The figure shows three views and two pictorial views of one solid part (mm, origin at its lowest corner). Answer the questions. A direction names the side the tool comes from. Round coordinates to 2 decimals unless told otherwise and drop trailing zeros. Order: outer loops, then holes, each group sorted by start corner. A loop starts at its lowest first (then second) coordinate and runs counter-clockwise, first axis right, second up. Notation, with made-up numbers: (26.5, 69.25) - (73.5, 69.25) arc R21 ccw to (73.5, 102.25) - close; hole circle Ø2 at (12, 81). An arc over 180 degrees is marked (long way). One line per item, written item: value. Start each with the question number.
1. Section C-C, the plane x = 17 is taken. Give the vertices of the cut face in (y, z), then the cut area to 3 significant figures.
2. Section D-D, the plane y = 12 is taken. Give the vertices of the cut face in (x, z).
3. For a pull along Y with two mould halves and no side action, classify the marked faces 3, 4, 5 and 6 as released by +Y, released by -Y, zero draft, split by the parting line, or undercut.
4. Flat-ended cylindrical pins translate along their axes: P1, Ø6, axis at x = 10, y = 7.5, coming from the +Z side; P2, Ø1.5, axis at y = 2.5, z = 7, coming from the +X side. Find the tip coordinate at first contact, or state that the pin passes through.
5. Section A-A, the plane z = 11 is taken. Give the vertices of the cut face in (x, y), then the cut area to 3 significant figures.
6. Straight lines are drawn through the part: line 1 (Y direction, x = 17.25, z = 20); line 2 (X direction, y = 4.75, z = 11); line 3 (X direction, y = 11.5, z = 9). For each, find the intervals that lie inside material, in ascending order.
7. Section B-B, the plane x = 11 is taken. Give the vertices of the cut face in (y, z), then the cut area to 3 significant figures.
8. A tool of negligible diameter and unlimited length cuts with its end or side. For the marked faces 1 and 2, from which of +Z, -Z, +X, -X, +Y, -Y can it reach the whole face along a straight path? Write none if from no direction.
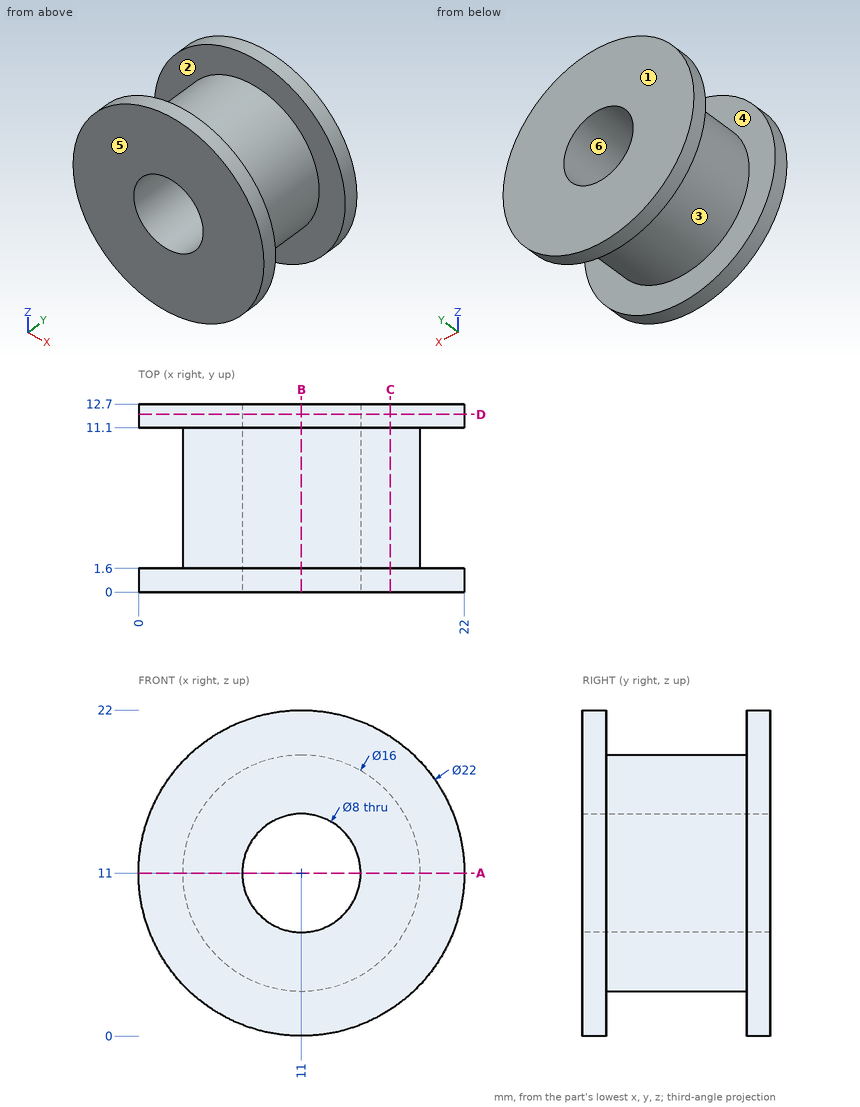
Answer list:
1. outline: (0, 1.78) - (1.6, 1.78) - (1.6, 5.71) - (11.1, 5.71) - (11.1, 1.78) - (12.7, 1.78) - (12.7, 20.22) - (11.1, 20.22) - (11.1, 16.29) - (1.6, 16.29) - (1.6, 20.22) - (0, 20.22) - close
1. area: 160 mm²
2. outline: circle Ø22 at (11, 11); hole circle Ø8 at (11, 11)
3. face 3: undercut
3. face 4: undercut
3. face 5: released by -Y
3. face 6: zero draft
4. P1: stops at z = 19
4. P2: stops at x = 18.31
5. outline: (0, 0) - (7, 0) - (7, 12.7) - (0, 12.7) - (0, 11.1) - (3, 11.1) - (3, 1.6) - (0, 1.6) - close; (15, 0) - (22, 0) - (22, 1.6) - (19, 1.6) - (19, 11.1) - (22, 11.1) - (22, 12.7) - (15, 12.7) - close
5. area: 121 mm²
6. line 1: y = 0 to 1.6, 11.1 to 12.7
6. line 2: x = 3 to 7, 15 to 19
6. line 3: x = 0.18 to 7.54, 14.46 to 21.82
7. outline: (0, 0) - (1.6, 0) - (1.6, 3) - (11.1, 3) - (11.1, 0) - (12.7, 0) - (12.7, 7) - (0, 7) - close; (0, 15) - (12.7, 15) - (12.7, 22) - (11.1, 22) - (11.1, 19) - (1.6, 19) - (1.6, 22) - (0, 22) - close
7. area: 121 mm²
8. face 1: +Z, -Z, +X, -X, +Y
8. face 2: none
